from build123d import *

# Parameters (mm, degrees)
SKETCH1_W                  = 110
SKETCH1_H                  = 90
BOSS_EXTRUDE1_DEPTH        = 7
M2_5_CLEARANCE_HOLE1_D     = 2.9
M2_5_CLEARANCE_HOLE1_DEPTH = 5
M2_5_CLEARANCE_HOLE1_TIP   = 0.871247898
SKETCH8_W                  = 5
SKETCH8_H                  = 20
CUT_EXTRUDE5_DEPTH         = 3
SKETCH10_W                 = 2
SKETCH10_H                 = 59.5
SKETCH10_H_2               = 10.5
CUT_EXTRUDE6_DEPTH         = 3
SKETCH11_W                 = 71
SKETCH11_H                 = 2
SKETCH11_W_2               = 17
CUT_EXTRUDE7_DEPTH         = 3
SKETCH12_W                 = 2
SKETCH12_H                 = 88
CUT_EXTRUDE8_DEPTH         = 3
SKETCH13_W                 = 106
SKETCH13_H                 = 2
CUT_EXTRUDE9_DEPTH         = 3
M2_5_CLEARANCE_HOLE2_D     = 2.9


with BuildPart() as part:
    # Sketch1 → Boss-Extrude1 (new body)
    with BuildSketch(Plane(origin=(0, 0, 0), x_dir=(1, 0, 0), z_dir=(0, 1, 0))):
        Rectangle(SKETCH1_W, SKETCH1_H)
    extrude(amount=BOSS_EXTRUDE1_DEPTH)

    # M2.5 Clearance Hole1
    with Locations(Plane(origin=(0, 7, 0), x_dir=(1, 0, 0), z_dir=(0, 1, 0))):
        with Locations((-31.5, 32), (13.5, 32), (31.5, -32)):
            Hole(M2_5_CLEARANCE_HOLE1_D / 2, depth=M2_5_CLEARANCE_HOLE1_DEPTH)
            with Locations((0, 0, -(M2_5_CLEARANCE_HOLE1_DEPTH + M2_5_CLEARANCE_HOLE1_TIP / 2))):  # 118° drill point
                Cone(0, M2_5_CLEARANCE_HOLE1_D / 2, M2_5_CLEARANCE_HOLE1_TIP, mode=Mode.SUBTRACT)

    # Sketch8 → Cut-Extrude5 (cut)
    with BuildSketch(Plane(origin=(0, 7, 0), x_dir=(1, 0, 0), z_dir=(0, 1, 0))):
        with Locations((-42.5, 0)):
            Rectangle(SKETCH8_W, SKETCH8_H)
        with Locations((42.5, 0)):
            Rectangle(SKETCH8_W, SKETCH8_H)
    extrude(amount=-CUT_EXTRUDE5_DEPTH, mode=Mode.SUBTRACT)

    # Sketch10 → Cut-Extrude6 (cut)
    with BuildSketch(Plane(origin=(0, 7, 0), x_dir=(1, 0, 0), z_dir=(0, 1, 0))):
        with Locations((-54, 15.25)):
            Rectangle(SKETCH10_W, SKETCH10_H)
        with Locations((-54, -39.75)):
            Rectangle(SKETCH10_W, SKETCH10_H_2)
    extrude(amount=-CUT_EXTRUDE6_DEPTH, mode=Mode.SUBTRACT)

    # Sketch11 → Cut-Extrude7 (cut)
    with BuildSketch(Plane(origin=(0, 7, 0), x_dir=(1, 0, 0), z_dir=(0, 1, 0))):
        with Locations((-17.5, 44)):
            Rectangle(SKETCH11_W, SKETCH11_H)
        with Locations((46.5, 44)):
            Rectangle(SKETCH11_W_2, SKETCH11_H)
    extrude(amount=-CUT_EXTRUDE7_DEPTH, mode=Mode.SUBTRACT)

    # Sketch12 → Cut-Extrude8 (cut)
    with BuildSketch(Plane(origin=(0, 7, 0), x_dir=(1, 0, 0), z_dir=(0, 1, 0))):
        with Locations((54, -1)):
            Rectangle(SKETCH12_W, SKETCH12_H)
    extrude(amount=-CUT_EXTRUDE8_DEPTH, mode=Mode.SUBTRACT)

    # Sketch13 → Cut-Extrude9 (cut)
    with BuildSketch(Plane(origin=(0, 7, 0), x_dir=(1, 0, 0), z_dir=(0, 1, 0))):
        with Locations((0, -44)):
            Rectangle(SKETCH13_W, SKETCH13_H)
    extrude(amount=-CUT_EXTRUDE9_DEPTH, mode=Mode.SUBTRACT)

    # M2.5 Clearance Hole2 (through all)
    with Locations(Plane(origin=(0, 7, 0), x_dir=(1, 0, 0), z_dir=(0, 1, 0))):
        with Locations((48.75, 38.75), (-48.75, 38.75), (48.75, -38.75), (-48.75, -38.75)):
            Hole(M2_5_CLEARANCE_HOLE2_D / 2)


solid = part.part
Input: part model. Units: mm. Frame: model coordinates. A direction names the side the tool comes from. Give positions to 0.01 mm unless a question says otherwise; leave off trailing zeros. Write each loop counter-clockwise with the first axis right and the second up, starting at its lowest first coordinate (ties: lowest second). Pieces come first, ordered by that corner, then holes.
Q1. Material intervals for probe 1 along X at (y, z) = (3.6, -32); probe 2 along X at (y, z) = (3.5, 38.75); probe 3 along Z at (x, y) = (48.75, 4.75), sorted ascending.
Q2. Pull-direction query (X, two-part tool) for faces 1 (the face through (-53, 6, -14)), 2 (the face through (31.25, 1.28, 31.99)), 3 (the face through (-1, 6, 43)); classes: pulls with the +X half, pulls with the -X half, needs draft (parallel to the pull), parting line crosses it, or undercut.
Q3. Section A-A, the plane z = -38.75. Output: boundary loops of the cut face in (x, y), plus the area to 3 significant figures.
Q4. Section B-B, the plane x = 48.75. Output: boundary loops of the cut face in (y, z).
Q5. Set-up query: faces 4 (the face through (42, 4, 0)), 5 (the face through (45, 6, -43)), 6 (the face through (49.9, 3.45, 39.63)), 7 (the face through (53, 6, 1)). Return all of +Z, -Z, +X, -X, +Y, -Y with unobstructed straight access to the full face (end or side cutting, diameter ignored); none if empty.
Q6. Section D-D, the plane z = -3. Output: boundary loops of the cut face in (x, y).
Q7. Section C-C, the plane x = -27. Output: boundary loops of the cut face in (y, z).
Q8. First-contact query: P1, Ø3.5, axis at x = 43.5, y = 6, coming from the +Z side; P2, Ø1.5, axis at y = 5.5, z = -0.5, coming from the +X side; P3, Ø3.5, axis at y = 6, z = -1.5, coming from the -X side. Flat tips, straight axial feed; report the tip coordinate or a pass-through.
Filled in:
1. probe 1: x = -55 to -32.95, -30.05 to 12.05, 14.95 to 55
1. probe 2: x = -55 to -50.2, -47.3 to 47.3, 50.2 to 55
1. probe 3: z = -43 to -40.2, -37.3 to 37.3, 40.2 to 43
2. face 1: pulls with the -X half
2. face 2: undercut
2. face 3: needs draft
3. outline: (-55, 0) - (-50.2, 0) - (-50.2, 7) - (-53, 7) - (-53, 4) - (-55, 4) - close; (-47.3, 0) - (47.3, 0) - (47.3, 7) - (-47.3, 7) - close; (50.2, 0) - (55, 0) - (55, 4) - (53, 4) - (53, 7) - (50.2, 7) - close
3. area: 717 mm2
4. outline: (0, -45) - (4, -45) - (4, -43) - (7, -43) - (7, -40.2) - (0, -40.2) - close; (0, -37.3) - (7, -37.3) - (7, 37.3) - (0, 37.3) - close; (0, 40.2) - (7, 40.2) - (7, 43) - (4, 43) - (4, 45) - (0, 45) - close
5. face 4: +Y
5. face 5: -Z, +X, +Y
5. face 6: +Y, -Y
5. face 7: +Z, -Z, +X, +Y
6. outline: (-55, 0) - (55, 0) - (55, 4) - (53, 4) - (53, 7) - (45, 7) - (45, 4) - (40, 4) - (40, 7) - (-40, 7) - (-40, 4) - (-45, 4) - (-45, 7) - (-53, 7) - (-53, 4) - (-55, 4) - close
7. outline: (0, -45) - (4, -45) - (4, -43) - (7, -43) - (7, 43) - (4, 43) - (4, 45) - (0, 45) - close
8. P1: stops at z = 43
8. P2: stops at x = 53
8. P3: stops at x = -53
